Design review of the part shown in the three views and the two pictorial views. Dimensions are in mm from the part's minimum x, y and z. A direction names the side the tool comes from. Give positions to 0.01 mm unless a question says otherwise; leave off trailing zeros. Loops run counter-clockwise (first coordinate to the right, second up) from the corner with the lowest first, then second, coordinate; pieces in that order, holes last.
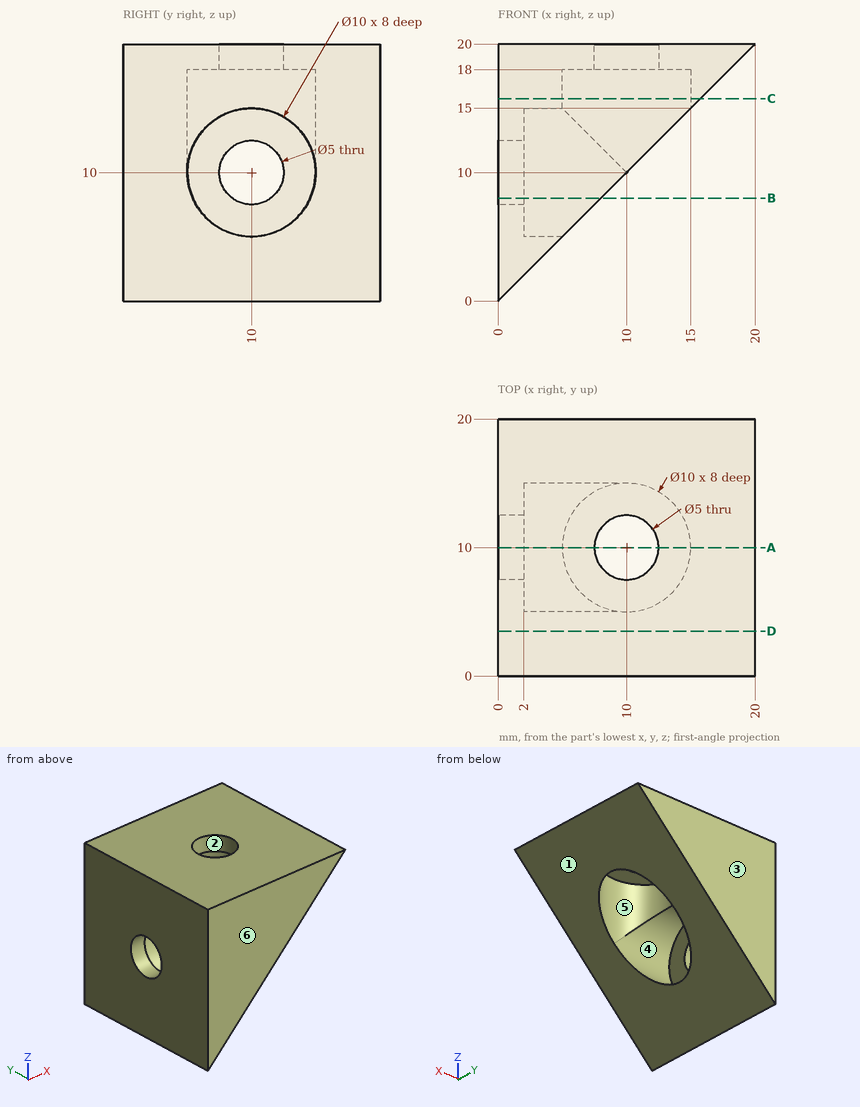
Q1. For probe 1 along Y at (x, z) = (6.75, 10); probe 2 along Y at (x, z) = (1.1, 10); probe 3 along X at (y, z) = (10.5, 5.5), list the stretches that pass through material, from the lowest coordinate up.
Answers:
probe 1: y = 0 to 5, 15 to 20
probe 2: y = 0 to 7.5, 12.5 to 20
probe 3: x = 0 to 2
Q2. Machinability: for the marked faces 4, 5 and 6, which of the approach directions +Z, -Z, +X, -X, +Y, -Y give a long, thin tool a straight path to every point of the face, cutting with its end or side? Answer none if there is none.
Answers:
face 4: +X
face 5: -Z
face 6: +Z, -Z, +X, -X, -Y
Q3. Consider section B-B on z = 8. Give the boundary of the cut face in (x, y).
Answers:
outline: (0, 0) - (8, 0) - (8, 5.42) - (2, 5.42) - (2, 8.5) - (0, 8.5) - close; (0, 11.5) - (2, 11.5) - (2, 14.58) - (8, 14.58) - (8, 20) - (0, 20) - close
Q4. Consider section A-A on y = 10. Give the boundary of the cut face in (x, z).
Answers:
outline: (0, 0) - (5, 5) - (2, 5) - (2, 7.5) - (0, 7.5) - close; (0, 12.5) - (2, 12.5) - (2, 15) - (5, 15) - (5, 18) - (7.5, 18) - (7.5, 20) - (0, 20) - close; (12.5, 18) - (15, 18) - (15, 15) - (20, 20) - (12.5, 20) - close
Q5. Mouldability with a two-part tool opening along Y and no side actions: class the marked faces 1, 2 and 3 as +Y half, -Y half, draft (parallel to the pull), parting line (faces both ways), or undercut.
Answers:
face 1: draft
face 2: undercut
face 3: +Y half
Q6. Consider section C-C on z = 15.75. Give the boundary of the cut face in (x, y).
Answers:
outline: (0, 0) - (15.75, 0) - (15.75, 20) - (0, 20) - close; hole circle Ø10 at (10, 10)
Q7. Consider section D-D on y = 3.5. Give the boundary of the cut face in (x, z), plus the area to 3 significant figures.
Answers:
outline: (0, 0) - (20, 20) - (0, 20) - close
area: 200 mm2
Q8. For pin 1 Ø1 at (x, z) = (14, 12) entering from -Y; pin 2 Ø5 at (y, z) = (16.5, 14) entering from +X; pin 3 Ø11.5 at (x, y) = (10, 10) entering from -Z; pin 4 Ø1.5 at (y, z) = (5, 8.5) entering from +X, all flat-tipped, find the tip position at first contact; note any pin that passes through.
Answers:
pin 1: passes through
pin 2: stops at x = 16.5
pin 3: stops at z = 4.25
pin 4: stops at x = 9.25
